Input: part model. Units: mm. Frame: model coordinates. Give positions to 0.01 mm unless a question says otherwise; leave off trailing zeros. Loops run counter-clockwise (first coordinate to the right, second up) from the corner with the lowest first, then second, coordinate; pieces in that order, holes last.
from build123d import *

# Parameters (mm, degrees)
SKETCH_1_R                       = 47.5
EXTRUDE_1_DEPTH                  = 1.5
CUT_EXTRUDE_1_DEPTH              = 68.191889392
CUT_EXTRUDE_2_DEPTH              = 68.191889392
CUT_EXTRUDE_2_DEPTH_BACK         = 68.191889392
SKETCH_3_R                       = 3.1
SKETCH_3_R_2                     = 1.6
SKETCH_4_R                       = 1.6
CUT_EXTRUDE_3_DEPTH              = 68.191889392
CUT_EXTRUDE_4_DEPTH              = 68.191889392
FILLET_1_R                       = 1
FILLET_2_R                       = 0.2
FILLET_3_R                       = 3.05
PATTERN_CIRCULAR_1_COUNT         = 8
FILLET_1_OF_PATTERN_CIRCULAR_1_R = 1
FILLET_2_OF_PATTERN_CIRCULAR_1_R = 0.2
FILLET_3_OF_PATTERN_CIRCULAR_1_R = 3.05
CUT_EXTRUDE_5_DEPTH              = 66.05834985
EXTRUDE_START                    = -1.5
EXTRUDE_2_DEPTH                  = 1.5
FILLET_4_R                       = 3.05
PATTERN_CIRCULAR_2_COUNT         = 8


with BuildPart() as part:
    # ｽｹｯﾁ1 → ﾎﾞｽ - 押し出し1 (new body)
    with BuildSketch(Plane.XY):
        Circle(SKETCH_1_R)
    extrude(amount=EXTRUDE_1_DEPTH)

    # ｽｹｯﾁ2 → ｶｯﾄ - 押し出し1 (cut, through all)
    with BuildSketch(Plane.XY.offset(1.5)):
        Polygon((-10.75, 43.525), (-10.75, 52.5), (10.75, 52.5), (10.75, 43.525), (13, 43.525), (13, 40.475), (10.75, 40.475), (10.75, 31.5), (-10.75, 31.5), (-10.75, 40.475), (-13, 40.475), (-13, 43.525), align=None)
    cut_extrude_1 = extrude(amount=-CUT_EXTRUDE_1_DEPTH, mode=Mode.SUBTRACT)

    # ｽｹｯﾁ3 → ｶｯﾄ - 押し出し2 (cut, two sides: drawn at the far end of the back side and taken through both)
    with BuildSketch(Plane.XY.offset(1.5).offset(-CUT_EXTRUDE_2_DEPTH_BACK)):
        Circle(SKETCH_3_R)
        with Locations((0, 6.5)):
            Circle(SKETCH_3_R_2)
        with Locations((6.5, 0)):
            Circle(SKETCH_3_R_2)
        with Locations((0, -6.5)):
            Circle(SKETCH_3_R_2)
        with Locations((-6.5, 0)):
            Circle(SKETCH_3_R_2)
        with Locations((8.838834765, 8.838834765)):
            Circle(SKETCH_3_R_2)
        with Locations((8.838834765, -8.838834765)):
            Circle(SKETCH_3_R_2)
        with Locations((-8.838834765, -8.838834765)):
            Circle(SKETCH_3_R_2)
        with Locations((-8.838834765, 8.838834765)):
            Circle(SKETCH_3_R_2)
    extrude(amount=CUT_EXTRUDE_2_DEPTH + CUT_EXTRUDE_2_DEPTH_BACK, mode=Mode.SUBTRACT)

    # ｽｹｯﾁ4 → ｶｯﾄ - 押し出し3 (cut, through all)
    with BuildSketch(Plane.XY.offset(1.5)):
        with Locations((14.733312146, 35.569362002)):
            Circle(SKETCH_4_R)
        with Locations((8.610377228, 20.787289482)):
            Circle(SKETCH_4_R)
    cut_extrude_3 = extrude(amount=-CUT_EXTRUDE_3_DEPTH, mode=Mode.SUBTRACT)

    # ｽｹｯﾁ5 → ｶｯﾄ - 押し出し4 (cut, symmetric)
    with BuildSketch(Plane.XY.offset(1.5)):
        Polygon((-7.188286702, 26.5), (7.188286702, 26.5), (3.328075632, 17.180626082), (-3.328075632, 17.180626082), align=None)
    cut_extrude_4 = extrude(amount=CUT_EXTRUDE_4_DEPTH, both=True, mode=Mode.SUBTRACT)

    # ﾌｨﾚｯﾄ1
    fillet_1_edges = [part.edges().sort_by_distance(p)[0] for p in [
        (7.188286702, 26.5, 0.75),
        (3.328075632, 17.180626082, 0.75),
        (-3.328075632, 17.180626082, 0.75),
        (-7.188286702, 26.5, 0.75),
        (10.75, 46.267564232, 0.75),
        (-10.75, 46.267564232, 0.75),
    ]]
    fillet(fillet_1_edges, radius=FILLET_1_R)

    # ﾌｨﾚｯﾄ2
    fillet_2_edges = [part.edges().sort_by_distance(p)[0] for p in [
        (13, 43.525, 0.75),
        (13, 40.475, 0.75),
        (-13, 40.475, 0.75),
        (-13, 43.525, 0.75),
    ]]
    fillet(fillet_2_edges, radius=FILLET_2_R)

    # ﾌｨﾚｯﾄ3
    fillet_3_edges = [part.edges().sort_by_distance(p)[0] for p in [
        (10.75, 31.5, 0.75),
        (-10.75, 31.5, 0.75),
    ]]
    fillet(fillet_3_edges, radius=FILLET_3_R)

    # 円形ﾊﾟﾀｰﾝ1: ｶｯﾄ - 押し出し1, ｶｯﾄ - 押し出し3, ｶｯﾄ - 押し出し4 ×8 about axis
    pattern_circular_1_axis = Axis((0, 0, 0), (0, 0, 1))
    add([cut_extrude_1.rotate(pattern_circular_1_axis, i * 360 / PATTERN_CIRCULAR_1_COUNT) for i in range(1, PATTERN_CIRCULAR_1_COUNT)], mode=Mode.SUBTRACT)
    add([cut_extrude_3.rotate(pattern_circular_1_axis, i * 360 / PATTERN_CIRCULAR_1_COUNT) for i in range(1, PATTERN_CIRCULAR_1_COUNT)], mode=Mode.SUBTRACT)
    add([cut_extrude_4.rotate(pattern_circular_1_axis, i * 360 / PATTERN_CIRCULAR_1_COUNT) for i in range(1, PATTERN_CIRCULAR_1_COUNT)], mode=Mode.SUBTRACT)

    # ﾌｨﾚｯﾄ1 of 円形ﾊﾟﾀｰﾝ1
    fillet_1_of_pattern_circular_1_edges = [part.edges().sort_by_distance(p)[0] for p in [
        (-13.655443429, 23.821215973, 0.75),
        (-9.79523236, 14.501842056, 0.75),
        (-14.501842056, 9.79523236, 0.75),
        (-23.821215973, 13.655443429, 0.75),
        (-25.11471052, 40.317506315, 0.75),
        (-40.317506315, 25.11471052, 0.75),
        (-26.5, 7.188286702, 0.75),
        (-17.180626082, 3.328075632, 0.75),
        (-17.180626082, -3.328075632, 0.75),
        (-26.5, -7.188286702, 0.75),
        (-46.267564232, 10.75, 0.75),
        (-46.267564232, -10.75, 0.75),
        (-23.821215973, -13.655443429, 0.75),
        (-14.501842056, -9.79523236, 0.75),
        (-9.79523236, -14.501842056, 0.75),
        (-13.655443429, -23.821215973, 0.75),
        (-40.317506315, -25.11471052, 0.75),
        (-25.11471052, -40.317506315, 0.75),
        (-7.188286702, -26.5, 0.75),
        (-3.328075632, -17.180626082, 0.75),
        (3.328075632, -17.180626082, 0.75),
        (7.188286702, -26.5, 0.75),
        (-10.75, -46.267564232, 0.75),
        (10.75, -46.267564232, 0.75),
        (13.655443429, -23.821215973, 0.75),
        (9.79523236, -14.501842056, 0.75),
        (14.501842056, -9.79523236, 0.75),
        (23.821215973, -13.655443429, 0.75),
        (25.11471052, -40.317506315, 0.75),
        (40.317506315, -25.11471052, 0.75),
        (26.5, -7.188286702, 0.75),
        (17.180626082, -3.328075632, 0.75),
        (17.180626082, 3.328075632, 0.75),
        (26.5, 7.188286702, 0.75),
        (46.267564232, -10.75, 0.75),
        (46.267564232, 10.75, 0.75),
        (23.821215973, 13.655443429, 0.75),
        (14.501842056, 9.79523236, 0.75),
        (9.79523236, 14.501842056, 0.75),
        (13.655443429, 23.821215973, 0.75),
        (40.317506315, 25.11471052, 0.75),
        (25.11471052, 40.317506315, 0.75),
    ]]
    fillet(fillet_1_of_pattern_circular_1_edges, radius=FILLET_1_OF_PATTERN_CIRCULAR_1_R)

    # ﾌｨﾚｯﾄ2 of 円形ﾊﾟﾀｰﾝ1
    fillet_2_of_pattern_circular_1_edges = [part.edges().sort_by_distance(p)[0] for p in [
        (-21.584434496, 39.969210807, 0.75),
        (-19.427758813, 37.812535124, 0.75),
        (-37.812535124, 19.427758813, 0.75),
        (-39.969210807, 21.584434496, 0.75),
        (-43.525, 13, 0.75),
        (-40.475, 13, 0.75),
        (-40.475, -13, 0.75),
        (-43.525, -13, 0.75),
        (-39.969210807, -21.584434496, 0.75),
        (-37.812535124, -19.427758813, 0.75),
        (-19.427758813, -37.812535124, 0.75),
        (-21.584434496, -39.969210807, 0.75),
        (-13, -43.525, 0.75),
        (-13, -40.475, 0.75),
        (13, -40.475, 0.75),
        (13, -43.525, 0.75),
        (21.584434496, -39.969210807, 0.75),
        (19.427758813, -37.812535124, 0.75),
        (37.812535124, -19.427758813, 0.75),
        (39.969210807, -21.584434496, 0.75),
        (43.525, -13, 0.75),
        (40.475, -13, 0.75),
        (40.475, 13, 0.75),
        (43.525, 13, 0.75),
        (39.969210807, 21.584434496, 0.75),
        (37.812535124, 19.427758813, 0.75),
        (19.427758813, 37.812535124, 0.75),
        (21.584434496, 39.969210807, 0.75),
    ]]
    fillet(fillet_2_of_pattern_circular_1_edges, radius=FILLET_2_OF_PATTERN_CIRCULAR_1_R)

    # ﾌｨﾚｯﾄ3 of 円形ﾊﾟﾀｰﾝ1
    fillet_3_of_pattern_circular_1_edges = [part.edges().sort_by_distance(p)[0] for p in [
        (-14.67246571, 29.875261505, 0.75),
        (-29.875261505, 14.67246571, 0.75),
        (-31.5, 10.75, 0.75),
        (-31.5, -10.75, 0.75),
        (-29.875261505, -14.67246571, 0.75),
        (-14.67246571, -29.875261505, 0.75),
        (-10.75, -31.5, 0.75),
        (10.75, -31.5, 0.75),
        (14.67246571, -29.875261505, 0.75),
        (29.875261505, -14.67246571, 0.75),
        (31.5, -10.75, 0.75),
        (31.5, 10.75, 0.75),
        (29.875261505, 14.67246571, 0.75),
        (14.67246571, 29.875261505, 0.75),
    ]]
    fillet(fillet_3_of_pattern_circular_1_edges, radius=FILLET_3_OF_PATTERN_CIRCULAR_1_R)

    # ｽｹｯﾁ6 → ｶｯﾄ - 押し出し5 (cut, through all)
    with BuildSketch(Plane.XY.offset(1.5)):
        Polygon((11.664524887, 28.160654182), (7.7, 28.5), (-7.7, 28.5), (-11.664524887, 28.160654182), (-14.707821049, 25.597265479), (-25.597265479, 14.707821049), (-28.160654182, 11.664524887), (-28.5, 7.7), (-28.5, -7.7), (-28.160654182, -11.664524887), (-25.597265479, -14.707821049), (-14.707821049, -25.597265479), (-11.664524887, -28.160654182), (-7.7, -28.5), (7.7, -28.5), (11.664524887, -28.160654182), (14.707821049, -25.597265479), (25.597265479, -14.707821049), (28.160654182, -11.664524887), (28.5, -7.7), (28.5, 7.7), (28.160654182, 11.664524887), (25.597265479, 14.707821049), (14.707821049, 25.597265479), align=None)
    extrude(amount=-CUT_EXTRUDE_5_DEPTH, mode=Mode.SUBTRACT)

    # ｽｹｯﾁ7 → ﾎﾞｽ - 押し出し2 (add)
    with BuildSketch(Plane.XY.offset(1.5).offset(EXTRUDE_START)):
        with BuildLine():
            Line((-12.8, 43.525), (-10.75, 43.525))
            Line((-10.75, 43.525), (-10.75, 40.475))
            Line((-10.75, 40.475), (-12.8, 40.475))
            ThreePointArc((-12.8, 40.475), (-12.941421356, 40.533578644), (-13, 40.675))
            Line((-13, 40.675), (-13, 43.325))
            ThreePointArc((-13, 43.325), (-12.941421356, 43.466421356), (-12.8, 43.525))
        make_face()
        with BuildLine():
            Line((12.8, 40.475), (10.75, 40.475))
            Line((10.75, 40.475), (10.75, 43.525))
            Line((10.75, 43.525), (12.8, 43.525))
            ThreePointArc((12.8, 43.525), (12.941421356, 43.466421356), (13, 43.325))
            Line((13, 43.325), (13, 40.675))
            ThreePointArc((13, 40.675), (12.941421356, 40.533578644), (12.8, 40.475))
        make_face()
    extrude_2 = extrude(amount=EXTRUDE_2_DEPTH)

    # ﾌｨﾚｯﾄ4
    fillet_4_edges = [part.edges().sort_by_distance(p)[0] for p in [
        (-11.664524887, 28.160654182, 0.75),
        (11.664524887, 28.160654182, 0.75),
        (28.160654182, 11.664524887, 0.75),
        (28.160654182, -11.664524887, 0.75),
        (11.664524887, -28.160654182, 0.75),
        (-11.664524887, -28.160654182, 0.75),
        (-28.160654182, -11.664524887, 0.75),
        (-28.160654182, 11.664524887, 0.75),
    ]]
    fillet(fillet_4_edges, radius=FILLET_4_R)

    # 円形ﾊﾟﾀｰﾝ2: ﾎﾞｽ - 押し出し2 ×8 about axis
    pattern_circular_2_axis = Axis((0, 0, 0), (0, 0, 1))
    for i in range(1, PATTERN_CIRCULAR_2_COUNT):
        add(extrude_2.rotate(pattern_circular_2_axis, i * 360 / PATTERN_CIRCULAR_2_COUNT))


solid = part.part
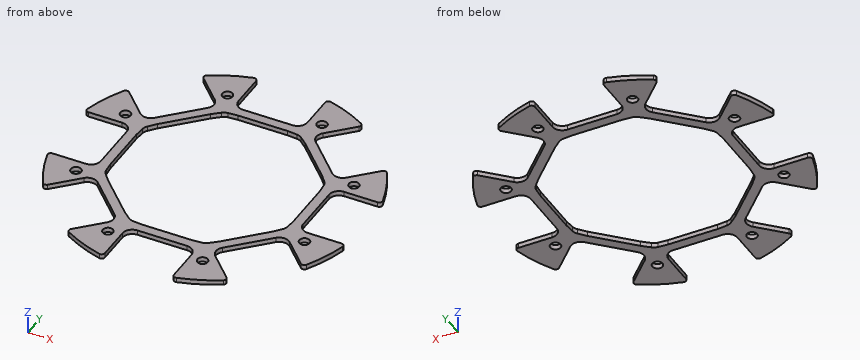
(1) Cut plane C-C (x = 22). Return the cut outline in (y, z).
Values follow:
outline: (-42.1, 0) - (-37.2, 0) - (-37.2, 1.5) - (-42.1, 1.5) - close; (-22.55, 0) - (-18.31, 0) - (-18.31, 1.5) - (-22.55, 1.5) - close; (18.31, 0) - (22.55, 0) - (22.55, 1.5) - (18.31, 1.5) - close; (37.2, 0) - (42.1, 0) - (42.1, 1.5) - (37.2, 1.5) - close
(2) Cut plane A-A (x = 6). Return the cut outline in (y, z), and give its area (3 significant figures).
Values follow:
outline: (-31.5, 0) - (-28.5, 0) - (-28.5, 1.5) - (-31.5, 1.5) - close; (28.5, 0) - (31.5, 0) - (31.5, 1.5) - (28.5, 1.5) - close
area: 9.00 mm2
(3) Pin query (flat end, axial travel): pin 1 Ø1.9 at (x, y) = (-35.57, -14.73) entering from -Z; pin 2 Ø0.8 at (y, z) = (4, 1) entering from -X; pin 3 Ø0.8 at (x, z) = (0.5, 1) entering from +Y. Return the tip coordinate at first contact, or that it passes through.
Values follow:
pin 1: passes through
pin 2: stops at x = -31.5
pin 3: stops at y = 31.5
(4) Cut plane D-D (z = 1). Count the separate pieces of the cut face and the enclosed holes in it, and give its area (3 significant figures).
Values follow:
separate pieces: 1
enclosed holes: 9
area: 1,690 mm2
(5) Ray query, probe 1 along Y at (x, z) = (-5.5, 0.55); probe 2 along X at (y, z) = (-14, 0.6); probe 3 along Y at (x, z) = (-17, 1.2). Return the intervals inside material, ascending.
Values follow:
probe 1: y = -31.5 to -28.5, 28.5 to 31.5
probe 2: x = -45.39 to -36.99, -34.15 to -26.19, 26.19 to 34.15, 36.99 to 45.39
probe 3: y = -44.35 to -32.2, -27.55 to -23.31, 23.31 to 27.55, 32.2 to 44.35
